The figure shows three views and two pictorial views of one solid part (mm, origin at its lowest corner). Answer the questions. Coordinates: 2 decimals unless noted, no trailing zeros. Write each loop counter-clockwise with the first axis right and the second up, starting at its lowest first coordinate (ties: lowest second). Pieces come first, ordered by that corner, then holes.
Item 1: A straight line is drawn through the part: probe 1 along Z at (x, y) = (58, 1.3). Find the intervals that lie inside material, in ascending order.
Item 2: Section B-B (y = 2.55) is taken. Give the vertices of the cut face in (x, z), then the cut area to 3 significant figures.
Item 3: Section A-A (z = 24.5) is taken. Give the vertices of the cut face in (x, y).
Item 4: Each of these flat-tipped pins is pushed along its axis until it touches: P1, Ø0.9, axis at y = 1.5, z = 2, coming from the -X side; P2, Ø0.9, axis at y = 1.5, z = 1.5, coming from the +X side; P3, Ø1.5, axis at x = 39.5, y = 1, coming from the -Z side. Where does it stop, or does it pass through?
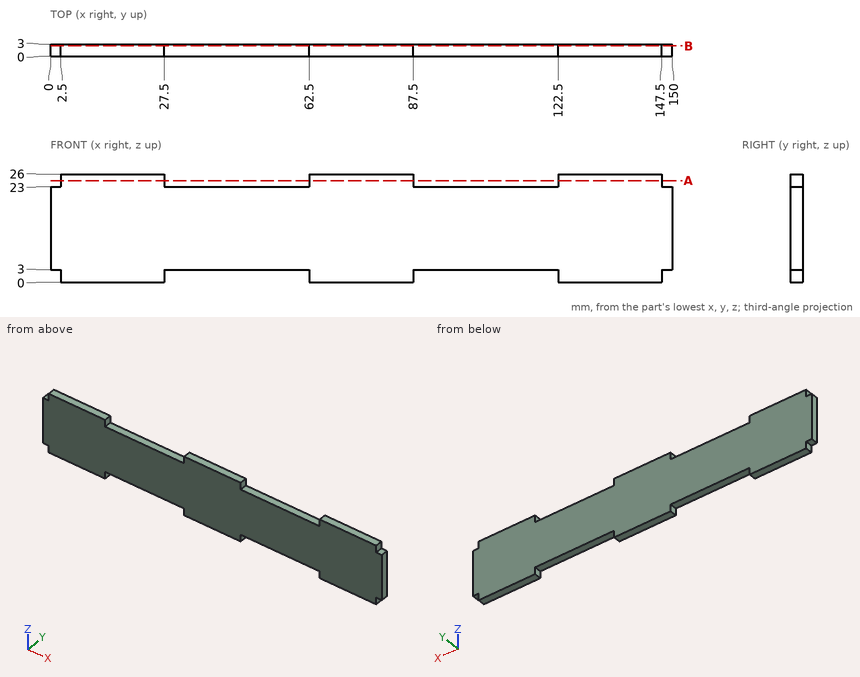
Established:
1. probe 1: z = 3 to 23
2. outline: (0, 3) - (2.5, 3) - (2.5, 0) - (27.5, 0) - (27.5, 3) - (62.5, 3) - (62.5, 0) - (87.5, 0) - (87.5, 3) - (122.5, 3) - (122.5, 0) - (147.5, 0) - (147.5, 3) - (150, 3) - (150, 23) - (147.5, 23) - (147.5, 26) - (122.5, 26) - (122.5, 23) - (87.5, 23) - (87.5, 26) - (62.5, 26) - (62.5, 23) - (27.5, 23) - (27.5, 26) - (2.5, 26) - (2.5, 23) - (0, 23) - close
2. area: 3,450 mm2
3. outline: (2.5, 0) - (27.5, 0) - (27.5, 3) - (2.5, 3) - close; (62.5, 0) - (87.5, 0) - (87.5, 3) - (62.5, 3) - close; (122.5, 0) - (147.5, 0) - (147.5, 3) - (122.5, 3) - close
4. P1: stops at x = 2.5
4. P2: stops at x = 147.5
4. P3: stops at z = 3
